Solid Edge part; units mm, degrees
sketch "Sketch1" plane through (0, 0, 0) normal (0, -1, 0) x (1, 0, 0)
  line L0 (-7.5, -7.5) -> (7.5, -7.5)
  line L1 (7.5, -7.5) -> (7.5, 7.5)
  line L2 (7.5, 7.5) -> (-7.5, 7.5)
  line L3 (-7.5, 7.5) -> (-7.5, -7.5)
  dimension "D1" = 7.5
  dimension "D2" = 7.5
extrude "Protrusion1" add sketch "Sketch1" against normal blind 25
sketch "Sketch2" plane through (0, 12.5, 7.5) normal (0, 0, 1) x (1, 0, 0)
  line L0 (-7.5, -12.5) -> (7.5, -12.5)
  line L1 (7.5, -12.5) -> (7.5, 4.5)
  line L2 (7.5, 4.5) -> (-7.5, 4.5)
  line L3 (-7.5, 4.5) -> (-7.5, -12.5)
  dimension "D1" = 7.5
extrude "Extrusionsausschnitt_1" cut sketch "Sketch2" against normal blind 7.5
fillet "Verrundung_1" radius 7.5 2 edges at (7.5, 0, -3.75) (-7.5, 0, -3.75)
sketch "Sketch3" plane through (0, 8.5, 0) normal (0, 0, 1) x (1, 0, 0)
  circle A0 centre (0, -1) radius 2.05
extrude "Cutout1" cut sketch "Sketch3" against normal through all
chamfer "Fase_1" distance 1 angle 45 2 edges at (-2.05, 7.5, 0) (2.05, 7.5, -7.5)
sketch "Sketch4" plane through (7.5, 16.25, 0) normal (1, 0, 0) x (0, 1, 0)
  line L0 (0.75, 7.5) -> (8.75, 7.5)
  line L1 (8.75, 7.5) -> (8.75, -7.5)
  line L2 (8.75, -7.5) -> (0.75, -7.5)
  line L3 (0.75, -7.5) -> (0.75, 7.5)
extrude "Extrusionsausprägung_2" add sketch "Sketch4" along normal blind 15
fillet "Verrundung_2" radius 7.5 2 edges at (22.5, 21, 7.5) (22.5, 21, -7.5)
sketch "Sketch5" plane through (7.5, 17, 0) normal (0, -1, 0) x (1, 0, 0)
  circle A0 centre (7.5, 0) radius 2.05
extrude "Cutout2" cut sketch "Sketch5" against normal through all
chamfer "Fase_2" distance 1 angle 45 2 edges at (12.95, 17, 0) (15, 25, 2.05)
fillet "Verrundung_3" radius 7.5 1 edges at (-7.5, 21, 7.5)
Design review of the part built by this model. Coordinates are the model's own, in mm. A direction names the side the tool comes from. Round coordinates to 2 decimals unless told otherwise and drop trailing zeros. Order: outer loops, then holes, each group sorted by start corner. A loop starts at its lowest first (then second) coordinate and runs counter-clockwise, first axis right, second up.
1) For L1, parallel to Z at x = 15, y = 19.55; L2, parallel to Y at x = 0, z = -4.65; L3, parallel to Y at x = 18.5, z = 2.5, list the stretches that pass through material, from the lowest coordinate up.
The answers:
L1: z = -7.5 to -2.05, 2.05 to 7.5
L2: y = 0 to 5.45, 9.55 to 25
L3: y = 17 to 25
2) Consider section B-B (x = 6.75). State the section outline as (y, z) points, plus the area to 3 significant figures.
The answers:
outline: (4.23, -7.5) - (25, -7.5) - (25, 7.5) - (17, 7.5) - (17, 0) - (4.23, 0) - close
area: 216 mm2
3) Draft analysis for pull direction Y (two halves, no side actions). For faces 4 (the cylindrical face through (-5.245, 2.138, -3.802)), 5 (the flat face through (8, 25, 0)), 6 (the flat face through (1, 15, -7.5)), 7 (the cylindrical face through (-0.444, 5.499, -3.712)), state which applies: released by +Y, released by -Y, zero draft, split by the parting line, or undercut.
The answers:
face 4: released by -Y
face 5: released by +Y
face 6: zero draft
face 7: undercut
4) Clearance check with flat-ended pins moving along their axes: pin 1 Ø10 at (x, y) = (15.5, 20) entering from +Z; pin 2 Ø4.5 at (x, y) = (0, 4.5) entering from +Z; pin 3 Ø4.5 at (x, z) = (11.5, 0.5) entering from -Y; pin 4 Ø2 at (y, z) = (14.5, -2.5) entering from +X. State where each tip first meets the part, or that it passes through.
The answers:
pin 1: stops at z = 7.5
pin 2: stops at z = 0
pin 3: stops at y = 17
pin 4: stops at x = 7.5
5) Machinability: for faces 1 (the flat face through (8, 17, 2)), 2 (the flat face through (7.5, 12, -4)), 3 (the flat face through (2, 11, 0)), which of the approach directions +Z, -Z, +X, -X, +Y, -Y give a long, thin tool a straight path to every point of the face, cutting with its end or side? Answer none if there is none.
The answers:
face 1: +Z, +X, -Y
face 2: +Z, -Z, +X, -Y
face 3: +Z, +X, -X, -Y
